Can you work these out from the model? Positions are in its coordinate system, mm. Face numbers are marked on the shaded views. A direction names the side the tool comes from. Coordinates: 2 decimals unless noted, no trailing zeros. Order: outer loops, then holes, each group sorted by start corner. A loop starts at its lowest first (then second) coordinate and runs counter-clockwise, first axis right, second up. Notation, with made-up numbers: (-13.5, 30) -> (39.5, 30) arc R17 ccw to (39.5, 54) -> close; hole circle Ø5 at (-16, 41.25). An arc over 180 degrees is marked (long way). Answer as CSV lines item,"result".
from build123d import *

# Parameters (mm, degrees)
BOSS_EXTRUDE1_DEPTH = 14
SKETCH1_3_R         = 20
SKETCH1_3_R_2       = 10
BOSS_EXTRUDE2_DEPTH = 20


with BuildPart() as part:
    # Sketch1 → Boss-Extrude1 (new body)
    with BuildSketch(Plane(origin=(0, 0, 0), x_dir=(1, 0, 0), z_dir=(0, 1, 0))):
        with BuildLine():
            ThreePointArc((48.282498705, -25.019990778), (34.462513349, -26.76164281), (27, -15))
            Line((27, -15), (27, 15))
            ThreePointArc((27, 15), (34.462513349, 26.76164281), (48.282498705, 25.019990778))
            ThreePointArc((48.282498705, 25.019990778), (30.821521428, 43.692867837), (18.665671202, 66.182807153))
            ThreePointArc((18.665671202, 66.182807153), (19.663588483, 62.652846559), (20, 59))
            ThreePointArc((20, 59), (-3.652846559, 39.336411517), (-18.665671202, 66.182807153))
            ThreePointArc((-18.665671202, 66.182807153), (-30.821521428, 43.692867837), (-48.282498705, 25.019990778))
            ThreePointArc((-48.282498705, 25.019990778), (-34.462513349, 26.76164281), (-27, 15))
            Line((-27, 15), (-27, -15))
            ThreePointArc((-27, -15), (-34.462513349, -26.76164281), (-48.282498705, -25.019990778))
            ThreePointArc((-48.282498705, -25.019990778), (-30.821521428, -43.692867837), (-18.665671202, -66.182807153))
            ThreePointArc((-18.665671202, -66.182807153), (-3.652846559, -39.336411517), (20, -59))
            ThreePointArc((20, -59), (19.663588483, -62.652846559), (18.665671202, -66.182807153))
            ThreePointArc((18.665671202, -66.182807153), (30.821521428, -43.692867837), (48.282498705, -25.019990778))
        make_face()
    extrude(amount=BOSS_EXTRUDE1_DEPTH)

    # Sketch1_3 → Boss-Extrude2 (add)
    # profile 1 of 4: a face of its own
    with BuildSketch(Plane(origin=(0, 0, 0), x_dir=(1, 0, 0), z_dir=(0, 1, 0))):
        with Locations(Location((0, -59, 0), (0, 0, 201.047411833))):
            Circle(SKETCH1_3_R)
        with Locations(Location((0, -59, 0), (0, 0, 270))):
            Circle(SKETCH1_3_R_2, mode=Mode.SUBTRACT)
    # profile 2 of 4: a face of its own
    with BuildSketch(Plane(origin=(0, 0, 0), x_dir=(1, 0, 0), z_dir=(0, 1, 0))):
        with BuildLine():
            Line((-53, -15), (-53, 15))
            ThreePointArc((-53, 15), (-40, 28), (-27, 15))
            Line((-27, 15), (-27, -15))
            ThreePointArc((-27, -15), (-40, -28), (-53, -15))
        make_face()
        with BuildLine():
            ThreePointArc((-32, 15), (-40, 23), (-48, 15))
            Line((-48, 15), (-48, -15))
            ThreePointArc((-48, -15), (-40, -23), (-32, -15))
            Line((-32, -15), (-32, 15))
        make_face(mode=Mode.SUBTRACT)
    # profile 3 of 4: a face of its own
    with BuildSketch(Plane(origin=(0, 0, 0), x_dir=(1, 0, 0), z_dir=(0, 1, 0))):
        with BuildLine():
            Line((27, -15), (27, 15))
            ThreePointArc((27, 15), (40, 28), (53, 15))
            Line((53, 15), (53, -15))
            ThreePointArc((53, -15), (40, -28), (27, -15))
        make_face()
        with BuildLine():
            ThreePointArc((48, 15), (40, 23), (32, 15))
            Line((32, 15), (32, -15))
            ThreePointArc((32, -15), (40, -23), (48, -15))
            Line((48, -15), (48, 15))
        make_face(mode=Mode.SUBTRACT)
    # profile 4 of 4: a face of its own
    with BuildSketch(Plane(origin=(0, 0, 0), x_dir=(1, 0, 0), z_dir=(0, 1, 0))):
        with Locations(Location((0, 59, 0), (0, 0, 21.047411833))):
            Circle(SKETCH1_3_R)
        with Locations(Location((0, 59, 0), (0, 0, 270))):
            Circle(SKETCH1_3_R_2, mode=Mode.SUBTRACT)
    extrude(amount=BOSS_EXTRUDE2_DEPTH)


solid = part.part
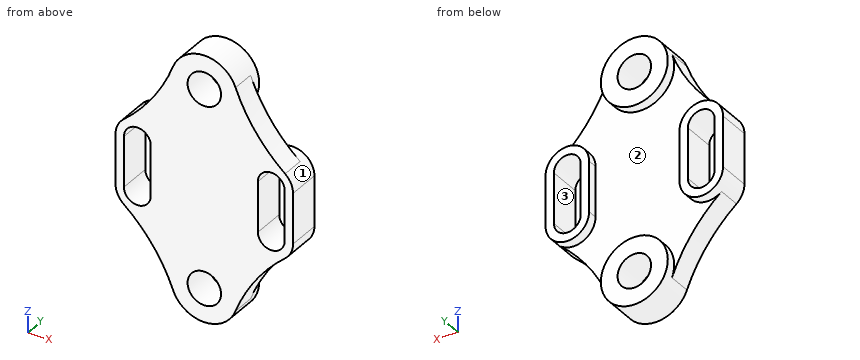
Q1. For P1, Ø1, axis at y = 11.5, z = 53.5, coming from the +X side; P2, Ø1.5, axis at x = 36.5, y = 9.5, coming from the +Z side; P3, Ø10, axis at y = 2.5, z = 45, coming from the +X side; P4, Ø3, axis at x = -6, z = 63, coming from the +Y side, each with a flat end and sliding along its axis, tell me the tip position at first contact or that it passes through.
Solution:
P1,"x = 24.88"
P2,"z = 37.39"
P3,"x = 33.61"
P4,"through"
Q2. If I drill on line 1 (X direction, y = 18.5, z = -7); line 2 (X direction, y = 9.5, z = 14); line 3 (X direction, y = 15.25, z = -19), over which ranges is the centre line in solid material (lowest first)?
Solution:
line 1,"-53 to -48, -32 to -27, 27 to 32, 48 to 53"
line 2,"-53 to -48, -32 to 32, 48 to 53"
line 3,"-52.37 to -46.93, -33.07 to -27.63, 27.63 to 33.07, 46.93 to 52.37"
Q3. Imagine slicing it at C-C (z = -59). List the corners of the cut face in (x, y) for me.
Solution:
outline,"(-21.76, 0) -> (-10, 0) -> (-10, 20) -> (-20, 20) -> (-20, 14) -> (-21.76, 14) -> close; (10, 0) -> (21.76, 0) -> (21.76, 14) -> (20, 14) -> (20, 20) -> (10, 20) -> close"
Q4. Imagine slicing it at A-A (x = 0). List the corners of the cut face in (y, z) for me, and give its area (3 significant figures).
Solution:
outline,"(0, -79) -> (20, -79) -> (20, -69) -> (0, -69) -> close; (0, -49) -> (20, -49) -> (20, -39) -> (14, -39) -> (14, 39) -> (20, 39) -> (20, 49) -> (0, 49) -> close; (0, 69) -> (20, 69) -> (20, 79) -> (0, 79) -> close"
area,"1,890 mm2"
Q5. Which directions (+Z, -Z, +X, -X, +Y, -Y) give clear straight access to the entire face, cutting with the end or side of a thin tool? Please do the marked faces 1, 2 and 3.
Solution:
face 1,"+Z, +Y"
face 2,"+Y"
face 3,"+Y, -Y"
Q6. Imagine slicing it at B-B (y = 10). List the corners of the cut face in (x, z) for me, and give its area (3 significant figures).
Solution:
outline,"(-53, -15) arc R13 ccw to (-48.28, -25.02) arc R100 cw to (-18.67, -66.18) arc R20 ccw to (18.67, -66.18) arc R100 cw to (48.28, -25.02) arc R13 ccw to (53, -15) -> (53, 15) arc R13 ccw to (48.28, 25.02) arc R100 cw to (18.67, 66.18) arc R20 ccw to (-18.67, 66.18) arc R100 cw to (-48.28, 25.02) arc R13 ccw to (-53, 15) -> close; hole (-48, -15) arc R8 ccw to (-32, -15) -> (-32, 15) arc R8 ccw to (-48, 15) -> close; hole circle Ø20 at (0, -59); hole circle Ø20 at (0, 59); hole (32, -15) arc R8 ccw to (48, -15) -> (48, 15) arc R8 ccw to (32, 15) -> close"
area,"9,020 mm2"
Q7. Imagine slicing it at D-D (x = 40.5). List the corners of the cut face in (y, z) for me.
Solution:
outline,"(0, -32.18) -> (14, -32.18) -> (14, -27.99) -> (20, -27.99) -> (20, -22.98) -> (0, -22.98) -> close; (0, 22.98) -> (20, 22.98) -> (20, 27.99) -> (14, 27.99) -> (14, 32.18) -> (0, 32.18) -> close"
